CAD build for the part. Positions are in the model's coordinates, mm. Face numbers are marked on the shaded views. Round coordinates to 2 decimals unless told otherwise and drop trailing zeros. Loops run counter-clockwise (first coordinate to the right, second up) from the corner with the lowest first, then second, coordinate; pieces in that order, holes last.
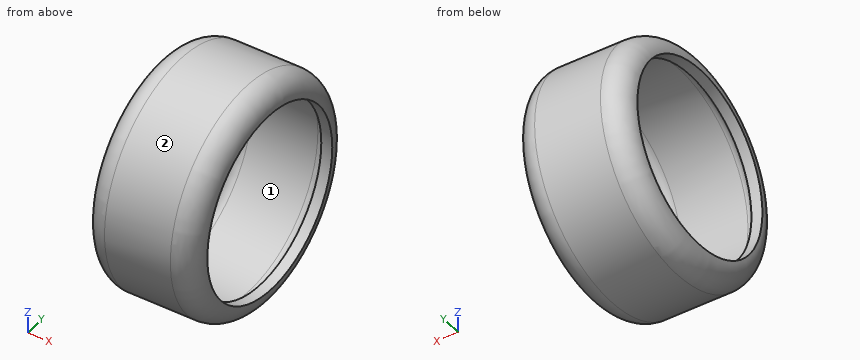
from build123d import *

# Parameters (mm, degrees)
F0_R     = 26.1896529573
F1_DEPTH = 25.4
F2_R     = 5.08
F3_T     = -2.54


# Not quite as in the source:
# - a shell that OpenCascade refuses in one call is made with other operations: the cavity is built on its own and cut out


with BuildPart() as f1:
    # F0 (on Right) → F1 (new body)
    with BuildSketch(Plane.YZ):
        with Locations((-9.9267605692, 26.3711642474)):
            Circle(F0_R)
    extrude(amount=F1_DEPTH)

    # F2
    f2_edges = [f1.edges().sort_by_distance(p)[0] for p in [
        (25.4, -36.116414, 26.371164),
        (0, -36.116414, 26.371164),
        (12.7, 16.262892, 26.371164),
    ]]
    fillet(f2_edges, radius=F2_R)

    # F3: a shell. OpenCascade refuses it in one call, so the cavity is built on its own and cut out:
    # the body offset inwards by the wall thickness, plus a prism from it out through each open face.
    f3_core = offset(f1.part, amount=F3_T, mode=Mode.PRIVATE)
    f3_exits = [f3_core.faces().sort_by_distance(p)[0] for p in [
        (22.86, -9.926761, 26.371164),
        (2.54, -9.926761, 26.371164),
    ]]
    add(f3_core, mode=Mode.SUBTRACT)
    extrude(f3_exits, amount=-F3_T, mode=Mode.SUBTRACT)


solid = f1.part
Item 1: Flat gauge pins, fed straight in: P1, Ø1, axis at x = 6, y = -22.5, coming from the +Z side; P2, Ø12, axis at x = 5.5, y = -29.5, coming from the +Z side; P3, Ø4, axis at x = 6.5, y = 7.5, coming from the +Z side. Where does each tip first touch, or does it go through?
Verdict:
P1: stops at z = 49.61
P2: stops at z = 48.77
P3: stops at z = 47.54
Item 2: Wall check: L1, parallel to X at y = -10.5, z = 5; L2, parallel to Y at x = 3.5, z = 21.5; L3, parallel to Y at x = 17, z = 11. Give the ranges that are in metal, low to high.
Verdict:
L1: x = 0.01 to 2.55, 22.85 to 25.39
L2: y = -35.4 to -32.51, 12.65 to 15.55
L3: y = -31.13 to -27.9, 8.05 to 11.28
Item 3: Mould opens along X. For the marked faces 1 and 2 say: released by +X, released by -X, zero draft, split by the parting line, or undercut.
Verdict:
face 1: undercut
face 2: zero draft
Item 4: Cut at A-A (x = 16.75). List the corners of the cut face in (y, z).
Verdict:
outline: circle Ø52.38 at (-9.93, 26.37); hole circle Ø47.3 at (-9.93, 26.37)
Item 5: Cut at B-B (x = 3.25). List the corners of the cut face in (y, z).
Verdict:
outline: circle Ø51.7 at (-9.93, 26.37); hole circle Ø45.74 at (-9.93, 26.37)
